```python
from build123d import *

# Parameters (mm, degrees)
ESQUISSE3_R             = 1.1
EXTRUSION1_DEPTH        = 9.5
ENL_V_MAT_EXTRU_2_DEPTH = 1.5
CHANFREIN1_SIZE         = 1.1
CHANFREIN1_SIZE2        = 1.905255888


with BuildPart() as part:
    # Esquisse1 → Révolution2 (revolve)
    with BuildSketch(Plane(origin=(0, 0, 0), x_dir=(0, 0, -1), z_dir=(1, 0, 0)), mode=Mode.PRIVATE) as r_volution2_sk:
        Polygon((0, 2.1), (1, 1.1), (1, 0), (0, 0), align=None)
    revolve(r_volution2_sk.sketch.rotate(Axis((0, 0, 1.603508429), (0, 0, -1)), 90), axis=Axis((0, 0, 1.603508429), (0, 0, -1)))

    # Esquisse3 → Extrusion1 (add)
    with BuildSketch(Plane.XY):
        Circle(ESQUISSE3_R)
    extrude(amount=-EXTRUSION1_DEPTH)

    # Esquisse2 → Enlèv. mat.-Extru.2 (cut)
    with BuildSketch(Plane.XY):
        Polygon((0, 0.808290377), (-0.7, 0.404145188), (-0.7, -0.404145188), (0, -0.808290377), (0.7, -0.404145188), (0.7, 0.404145188), align=None)
    extrude(amount=-ENL_V_MAT_EXTRU_2_DEPTH, mode=Mode.SUBTRACT)

    # Chanfrein1
    chanfrein1_edges = [part.edges().sort_by_distance(p)[0] for p in [
        (-1.1, 0, -9.5),
    ]]
    chanfrein1_side = [part.faces().sort_by_distance(p)[0] for p in [
        (0, 0, -9.5),
    ]]
    chamfer(chanfrein1_edges, length=CHANFREIN1_SIZE, length2=CHANFREIN1_SIZE2, reference=chanfrein1_side[0])


solid = part.part
```
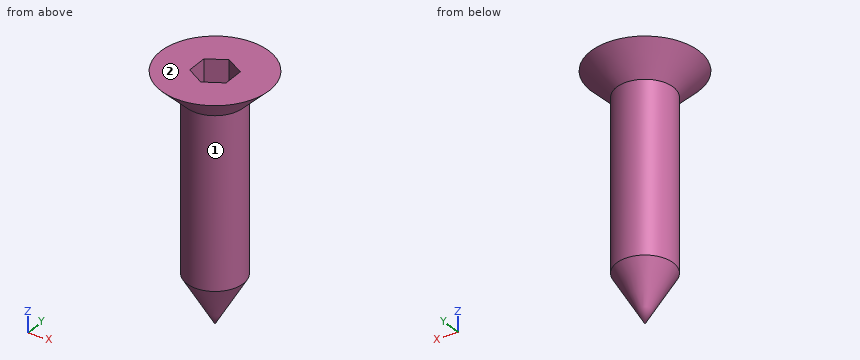
CAD build for the part. Positions are in the model's coordinates, mm. Face numbers are marked on the shaded views. A direction names the side the tool comes from. Round coordinates to 2 decimals unless told otherwise and drop trailing zeros. Order: outer loops, then holes, each group sorted by start corner. A loop starts at its lowest first (then second) coordinate and runs counter-clockwise, first axis right, second up.
Q1. Drop flat-ended pins along their axis: pin 1 (1.1 mm diameter, centred on x = 0, y = 0, fed in from +Z); pin 2 (1 mm diameter, centred on y = -1, z = -2, fed in from +X). Give the stop position or say it passes through.
Q2. Slice it at A-A (z = -1.25). Write the cut outline in (x, y).
Q3. Wall check: L1, parallel to Y at x = 0.65, z = -0.25; L2, parallel to Z at x = -0.75, y = -1.65; L3, parallel to Z at x = -1.6, y = -1.05. Give the ranges that are in metal, low to high.
Q4. Slice it at B-B (z = -7.5). Write the cut outline in (x, y), and give its area (3 significant figures).
Q5. Which spindle directions (+Z, -Z, +X, -X, +Y, -Y) get a long thin tool onto all of the face, cutting with end or side? Do the marked faces 1 and 2. Say none if no direction does.
Results below:
1. pin 1: stops at z = -1.5
1. pin 2: stops at x = 0.98
2. outline: circle Ø2.2 at (0, 0); hole (-0.7, -0.4) - (0, -0.81) - (0.7, -0.4) - (0.7, 0.4) - (0, 0.81) - (-0.7, 0.4) - close
3. L1: y = -1.73 to -0.43, 0.43 to 1.73
3. L2: z = -0.29 to 0
3. L3: z = -0.19 to 0
4. outline: circle Ø2.2 at (0, 0)
4. area: 3.80 mm2
5. face 1: -Z
5. face 2: +Z, +X, -X, +Y, -Y
